from build123d import *

# Parameters (mm, degrees)
CROQUIS1_R              = 2
CROQUIS1_R_2            = 10
SALIENTE_EXTRUIR1_DEPTH = 5
CROQUIS2_R              = 7.5
CROQUIS2_R_2            = 2.5
CROQUIS2_R_3            = 2
CORTAR_EXTRUIR1_DEPTH   = 10


with BuildPart() as part:
    # Croquis1 → Saliente-Extruir1 (new body)
    with BuildSketch(Plane(origin=(0, 0, 0), x_dir=(0, 0, -1), z_dir=(1, 0, 0))):
        with BuildLine():
            Line((10, 0), (60, 0))
            ThreePointArc((60, 0), (67.071067812, 2.928932188), (70, 10))
            Line((70, 10), (70, 60))
            ThreePointArc((70, 60), (67.071067812, 67.071067812), (60, 70))
            Line((60, 70), (60, 80))
            ThreePointArc((60, 80), (57.071067812, 87.071067812), (50, 90))
            Line((50, 90), (20, 90))
            ThreePointArc((20, 90), (12.928932188, 87.071067812), (10, 80))
            Line((10, 80), (10, 70))
            ThreePointArc((10, 70), (2.928932188, 67.071067812), (0, 60))
            Line((0, 60), (0, 10))
            ThreePointArc((0, 10), (2.928932188, 2.928932188), (10, 0))
        make_face()
        with Locations((7, 63)):
            Circle(CROQUIS1_R, mode=Mode.SUBTRACT)
        with Locations((63, 63)):
            Circle(CROQUIS1_R, mode=Mode.SUBTRACT)
        with Locations((63, 7)):
            Circle(CROQUIS1_R, mode=Mode.SUBTRACT)
        with Locations((7, 7)):
            Circle(CROQUIS1_R, mode=Mode.SUBTRACT)
        with Locations((35, 35)):
            Circle(CROQUIS1_R_2, mode=Mode.SUBTRACT)
    extrude(amount=SALIENTE_EXTRUIR1_DEPTH)

    # Croquis2 → Cortar-Extruir1 (cut)
    with BuildSketch(Plane(origin=(5, 0, 0), x_dir=(0, 0, -1), z_dir=(1, 0, 0))):
        with Locations((15, 0)):
            Circle(CROQUIS2_R)
        with Locations((50, 58)):
            Circle(CROQUIS2_R_2)
        with Locations((52, 83)):
            Circle(CROQUIS2_R_3)
        with Locations((34, 83)):
            Circle(CROQUIS2_R_3)
    extrude(amount=-CORTAR_EXTRUIR1_DEPTH, mode=Mode.SUBTRACT)


solid = part.part
The listing builds one solid part. Answer for the finished solid, in the listing's coordinates (mm). Coordinates: 2 decimals unless noted, no trailing zeros. Loops run counter-clockwise (first coordinate to the right, second up) from the corner with the lowest first, then second, coordinate; pieces in that order, holes last. Notation, with made-up numbers: (-20, 57.5) -> (24, 57.5) arc R35 cw to (24, 96.5) -> close; hole circle Ø7 at (22.25, 48). An arc over 180 degrees is marked (long way). Answer in a Markdown table with one row per item. Add a question column.
1. Consider line 1 (Y direction, x = 3.3, z = -35); line 2 (Y direction, x = 1.55, z = -7); line 3 (Z direction, x = 3.75, y = 42). Determine where each line is inside the solid, lowest interval first. Write a range as [from, to].
2. The part is cut by section B-B, the plane y = 58. Write down the section's boundary in (x, z).
3. The part is cut by section A-A, the plane x = 1.45. Count the separate pieces of the cut face and the enclosed holes in it, then the cut area to 3 significant figures.
4. The part is cut by section D-D, the plane y = 83. Write down the section's boundary in (x, z).
5. Flat-ended cylindrical pins translate along their axes: P1, Ø12, axis at y = 20, z = -20, coming from the -X side; P2, Ø3.5, axis at y = 63, z = -63, coming from the +X side; P3, Ø1, axis at x = 1.5, y = 62, coming from the -Z side. Find the tip coordinate at first contact, or state that the pin passes through.
6. The part is cut by section C-C, the plane z = -34. Write down the section's boundary in (x, y), then the cut area to 3 significant figures.
7. Determine the mould class of faces 1 (the flat face through (0, 46, -35)), 2 (the flat face through (2, 75, -10)), 3 (the cylindrical face through (2.46, 25.24, -32.83)) for opening direction Z: +Z half, -Z half, draft (parallel to the pull), parting line (faces both ways), or undercut.
Answer below:
| question | item | result |
|---|---|---|
| 1 | line 1 | [0, 25], [45, 81.27], [84.73, 90] |
| 1 | line 2 | [0.46, 5], [9, 61], [65, 69.54] |
| 1 | line 3 | [-70, -42.14], [-27.86, 0] |
| 2 | outline | (0, -70) -> (5, -70) -> (5, -52.5) -> (0, -52.5) -> close; (0, -47.5) -> (5, -47.5) -> (5, 0) -> (0, 0) -> close |
| 3 | separate pieces | 1 |
| 3 | enclosed holes | 8 |
| 3 | area | 5,270 mm2 |
| 4 | outline | (0, -59.54) -> (5, -59.54) -> (5, -54) -> (0, -54) -> close; (0, -50) -> (5, -50) -> (5, -36) -> (0, -36) -> close; (0, -32) -> (5, -32) -> (5, -10.46) -> (0, -10.46) -> close |
| 5 | P1 | x = 0 |
| 5 | P2 | through |
| 5 | P3 | z = -69.89 |
| 6 | outline | (0, 0) -> (5, 0) -> (5, 25.05) -> (0, 25.05) -> close; (0, 44.95) -> (5, 44.95) -> (5, 81) -> (0, 81) -> close; (0, 85) -> (5, 85) -> (5, 90) -> (0, 90) -> close |
| 6 | area | 331 mm2 |
| 7 | face 1 | draft |
| 7 | face 2 | +Z half |
| 7 | face 3 | undercut |
